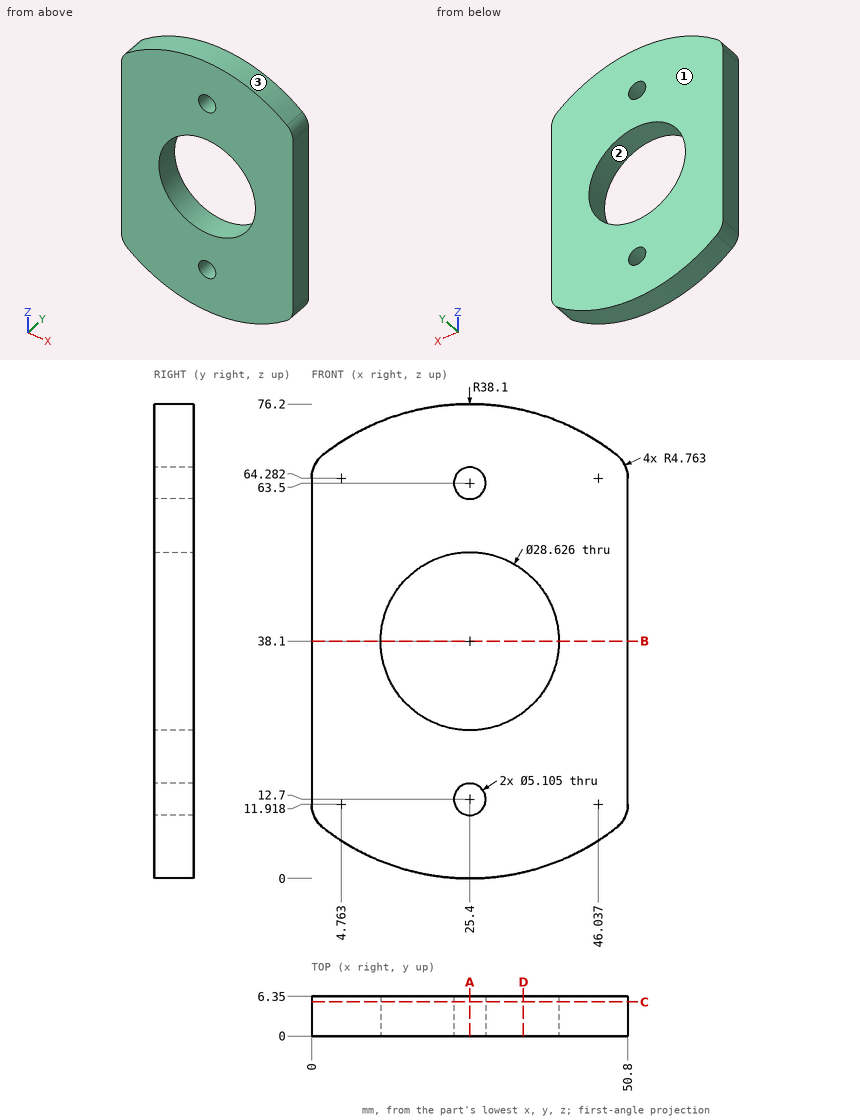
Design review of the part shown in the three views and the two pictorial views. Dimensions are in mm from the part's minimum x, y and z. Coordinates: 2 decimals unless noted, no trailing zeros. Loops run counter-clockwise (first coordinate to the right, second up) from the corner with the lowest first, then second, coordinate; pieces in that order, holes last.
Q1. We need section B-B on z = 38.1. State the section outline as (x, y) points.
Reported:
outline: (0, 0) - (11.09, 0) - (11.09, 6.35) - (0, 6.35) - close; (39.71, 0) - (50.8, 0) - (50.8, 6.35) - (39.71, 6.35) - close
Q2. To check wall thickness, follow line 1 (X direction, y = 2, z = 38); line 2 (Z direction, x = 27, y = 3) (1 decimal); line 3 (Z direction, x = 31.5, y = 5.75). State the ranges of each line that lie inside material, in increasing order.
Reported:
line 1: x = 0 to 11.09, 39.71 to 50.8
line 2: z = 0 to 10.7, 14.7 to 23.9, 52.3 to 61.5, 65.5 to 76.2
line 3: z = 0.49 to 25.15, 51.05 to 75.71
Q3. We need section C-C on y = 5.5. State the section outline as (x, z) points (1 decimal), and give its area (3 significant figures).
Reported:
outline: (0, 11.9) arc R4.8 ccw to (1.8, 8.2) arc R38.1 ccw to (49, 8.2) arc R4.8 ccw to (50.8, 11.9) - (50.8, 64.3) arc R4.8 ccw to (49, 68) arc R38.1 ccw to (1.8, 68) arc R4.8 ccw to (0, 64.3) - close; hole circle Ø28.6 at (25.4, 38.1); hole circle Ø5.1 at (25.4, 12.7); hole circle Ø5.1 at (25.4, 63.5)
area: 2,870 mm2
Q4. We need section D-D on x = 34. State the section outline as (y, z) points, and give its area (3 significant figures).
Reported:
outline: (0, 0.98) - (6.35, 0.98) - (6.35, 26.66) - (0, 26.66) - close; (0, 49.54) - (6.35, 49.54) - (6.35, 75.22) - (0, 75.22) - close
area: 326 mm2
Q5. We need section A-A on x = 25.4. State the section outline as (y, z) points, and give its area (3 significant figures).
Reported:
outline: (0, 0) - (6.35, 0) - (6.35, 10.15) - (0, 10.15) - close; (0, 15.25) - (6.35, 15.25) - (6.35, 23.79) - (0, 23.79) - close; (0, 52.41) - (6.35, 52.41) - (6.35, 60.95) - (0, 60.95) - close; (0, 66.05) - (6.35, 66.05) - (6.35, 76.2) - (0, 76.2) - close
area: 237 mm2
Q6. For pin 1 (1.5 mm diameter, centred on x = 7.5, y = 3.5, fed in from -Z); pin 2 (3 mm diameter, centred on y = 2.5, z = 67.5, fed in from +X), all flat-tipped, find the tip position at first contact; note any pin that passes through.
Reported:
pin 1: stops at z = 4.08
pin 2: stops at x = 50.48
Q7. The part is to be moulded in two halves that separate along X. For the marked faces 1, 2 and 3, say which applies: +X half, -X half, draft (parallel to the pull), parting line (faces both ways), or undercut.
Reported:
face 1: draft
face 2: undercut
face 3: parting line
